from build123d import *

# Parameters (mm, degrees)
SKETCH1_W           = 25
SKETCH1_H           = 60
BOSS_EXTRUDE1_DEPTH = 60
SKETCH2_W           = 30
SKETCH2_H           = 10
BOSS_EXTRUDE2_DEPTH = 10
SKETCH3_R           = 1.6
CUT_EXTRUDE1_DEPTH  = 83.764726786
FILLET3_R           = 5


with BuildPart() as part:
    # Sketch1 → Boss-Extrude1 (new body)
    with BuildSketch(Plane(origin=(0, 0, 0), x_dir=(1, 0, 0), z_dir=(0, 1, 0))):
        with Locations((12.5, 30)):
            Rectangle(SKETCH1_W, SKETCH1_H)
    extrude(amount=BOSS_EXTRUDE1_DEPTH)

    # Sketch2 → Boss-Extrude2 (add)
    with BuildSketch(Plane(origin=(25, 0, 0), x_dir=(0, 0, -1), z_dir=(1, 0, 0))):
        with Locations((30, 7)):
            Rectangle(SKETCH2_W, SKETCH2_H)
    extrude(amount=BOSS_EXTRUDE2_DEPTH)

    # Sketch3 → Cut-Extrude1 (cut, through all)
    with BuildSketch(Plane(origin=(0, 0, -45), x_dir=(-1, 0, 0), z_dir=(0, 0, -1))):
        with Locations((-30, 7)):
            Circle(SKETCH3_R)
    extrude(amount=-CUT_EXTRUDE1_DEPTH, mode=Mode.SUBTRACT)

    # Fillet3
    fillet3_edges = [part.edges().sort_by_distance(p)[0] for p in [
        (35, 2, -30),
        (35, 12, -30),
    ]]
    fillet(fillet3_edges, radius=FILLET3_R - 0.0001)  # a hair under: the kernel refuses the full size


solid = part.part
Work out the finished part from the listing and answer in its coordinate system (mm). A direction names the side the tool comes from. Give positions to 0.01 mm unless a question says otherwise; leave off trailing zeros. Order: outer loops, then holes, each group sorted by start corner. A loop starts at its lowest first (then second) coordinate and runs counter-clockwise, first axis right, second up. Notation, with made-up numbers: (-6.5, -33.75) -> (25.5, -33.75) arc R8 cw to (25.5, -29.75) -> close; hole circle Ø2 at (58.25, 2). An arc over 180 degrees is marked (long way). Answer as a JSON object with one key per item and string values. Group by question number.
1. Consider line 1 along Y through (x, z) = (30, -30.5); line 2 along X through (y, z) = (38, -54.5); line 3 along Y through (x, z) = (33, -32.5). Determine where each line is inside the solid, lowest interval first. Write a range as [from, to].
2. Section D-D on y = 39 is taken. Determine the outline of the cut face in (x, z), plus the area to 3 significant figures.
3. Section B-B on y = 9.5 is taken. Determine the outline of the cut face in (x, z), plus the area to 3 significant figures.
4. Flat-ended cylindrical pins translate along their axes: pin 1 Ø2.5 at (x, y) = (30, 7) entering from -Z; pin 2 Ø11 at (x, y) = (32.5, 6) entering from +Z; pin 3 Ø5 at (x, y) = (31, 9) entering from -Z. Find the tip coordinate at first contact, or state that the pin passes through.
5. Section C-C on z = -5 is taken. Determine the outline of the cut face in (x, y), plus the area to 3 significant figures.
6. A tool of negligible diameter and unlimited length cuts with its end or side. For faces 5 (the flat face through (27, 12, -30)), 6 (the flat face through (28, 7, -15)), 7 (the flat face through (28, 7, -45)), from which of +Z, -Z, +X, -X, +Y, -Y can it reach the whole face along a straight path? Write none if from no direction.
7. The mould has two halves that part along X. Classify faces 1 (the cylindrical face through (33, 11, -30)), 2 (the flat face through (27, 2, -30)), 3 (the cylindrical face through (31.27, 6.03, -30.21)), 4 (the flat face through (0, 30, -30)): released by +X, released by -X, zero draft, split by the parting line, or undercut.
Result sheet:
{
 "1": {"line 1": "y = [2, 5.4], [8.6, 12]", "line 2": "x = [0, 25]", "line 3": "y = [3, 11]"},
 "2": {"outline": "(0, -60) -> (25, -60) -> (25, 0) -> (0, 0) -> close", "area": "1,500 mm^2"},
 "3": {"outline": "(0, -60) -> (25, -60) -> (25, -45) -> (34.33, -45) -> (34.33, -15) -> (25, -15) -> (25, 0) -> (0, 0) -> close", "area": "1,780 mm^2"},
 "4": {"pin 1": "passes through", "pin 2": "stops at z = -15", "pin 3": "stops at z = -45"},
 "5": {"outline": "(0, 0) -> (25, 0) -> (25, 60) -> (0, 60) -> close", "area": "1,500 mm^2"},
 "6": {"face 5": "+Z, -Z, +X, +Y", "face 6": "+Z, +X, +Y, -Y", "face 7": "-Z, +X, +Y, -Y"},
 "7": {"face 1": "released by +X", "face 2": "zero draft", "face 3": "undercut", "face 4": "released by -X"}
}
